Read the model definition and answer for the solid it produces. Units are mm, in the model's axes. A direction names the side the tool comes from. Give positions to 0.01 mm unless a question says otherwise; leave off trailing zeros. Order: outer loops, then holes, each group sorted by start corner. A loop starts at its lowest first (then second) coordinate and runs counter-clockwise, first axis right, second up. Notation, with made-up numbers: (66.5, 39.5) - (94.5, 39.5) arc R21 ccw to (94.5, 45.5) - close; hole circle Ø2 at (-25.5, 81). An arc over 180 degrees is marked (long way). Answer as CSV lines item,"result". Start each with the question number.
from build123d import *

# Parameters (mm, degrees)
SKETCH1_W           = 62.4
SKETCH1_H           = 72.5
SKETCH1_W_2         = 2.8
SKETCH1_H_2         = 33.45
BOSS_EXTRUDE1_DEPTH = 2.8
CUT_EXTRUDE1_DEPTH  = 3.8


with BuildPart() as part:
    # Sketch1 → Boss-Extrude1 (new body)
    with BuildSketch(Plane.XY):
        with Locations((25.4, 22.394209189)):
            Rectangle(SKETCH1_W, SKETCH1_H)
        with Locations((-1.4, 5.669209189)):
            Rectangle(SKETCH1_W_2, SKETCH1_H_2, mode=Mode.SUBTRACT)
        with Locations((52.2, 5.669209189)):
            Rectangle(SKETCH1_W_2, SKETCH1_H_2, mode=Mode.SUBTRACT)
    extrude(amount=BOSS_EXTRUDE1_DEPTH)

    # Sketch2 → Cut-Extrude1 (cut, through all)
    with BuildSketch(Plane.XY.offset(2.8)):
        Polygon((0, -11.055790811), (-1.8, -11.055790811), (-1.8, -12.055790811), (-2.8, -13.055790811), (-2.8, -13.855790811), (0, -13.855790811), align=None)
    cut_extrude1 = extrude(amount=-CUT_EXTRUDE1_DEPTH, mode=Mode.SUBTRACT)

    # Mirror1: Cut-Extrude1 across plane
    add(cut_extrude1.mirror(Plane.ZY.offset(-25.4)), mode=Mode.SUBTRACT)


solid = part.part
(1) Which of the six approach directions +Z, -Z, +X, -X, +Y, -Y give full straight-line access (tool end or side, diameter ignored) to faces 1 (the flat face through (0, 4, 1)), 2 (the flat face through (25, -13.856, 1)), 3 (the flat face through (53.6, 5, 1))?
(2) Section B-B, the plane z = 0.95 is taken. Write down the section's boundary in (x, y).
(3) Straight lines are drawn through the part: line 1 (X direction, y = 18, z = 1); line 2 (Y direction, x = -1, z = 2.65); line 3 (Y direction, x = 53.5, z = 1.6). For each, find the intervals that lie inside material, in ascending order. Write a range as [from, to].
(4) Section A-A, the plane y = -2.5 is taken. Write down the section's boundary in (x, z), and give its area (3 significant figures).
(5) Determine the mould class of faces 4 (the flat face through (25, 58.644, 1)), 5 (the flat face through (52, 22.394, 1)), 6 (the flat face through (56.6, 22, 1)) for opening direction X: released by +X, released by -X, zero draft, split by the parting line, or undercut.
Checks:
1,face 1,"+Z, -Z, -Y"
1,face 2,"+Z, -Z, +X, -X, -Y"
1,face 3,"+Z, -Z"
2,outline,"(-5.8, -13.86) - (-2.8, -13.86) - (-2.8, -13.06) - (-1.8, -12.06) - (-1.8, -11.06) - (-2.8, -11.06) - (-2.8, 22.39) - (0, 22.39) - (0, -13.86) - (50.8, -13.86) - (50.8, 22.39) - (53.6, 22.39) - (53.6, -11.06) - (52.6, -11.06) - (52.6, -12.06) - (53.6, -13.06) - (53.6, -13.86) - (56.6, -13.86) - (56.6, 58.64) - (-5.8, 58.64) - close"
3,line 1,"x = [-5.8, -2.8], [0, 50.8], [53.6, 56.6]"
3,line 2,"y = [22.39, 58.64]"
3,line 3,"y = [-12.96, -11.06], [22.39, 58.64]"
4,outline,"(-5.8, 0) - (-2.8, 0) - (-2.8, 2.8) - (-5.8, 2.8) - close; (0, 0) - (50.8, 0) - (50.8, 2.8) - (0, 2.8) - close; (53.6, 0) - (56.6, 0) - (56.6, 2.8) - (53.6, 2.8) - close"
4,area,"159 mm²"
5,face 4,"zero draft"
5,face 5,"undercut"
5,face 6,"released by +X"
